Design review of the part built by this model. Coordinates are the model's own, in mm. Face numbers are marked on the shaded views. A direction names the side the tool comes from. Coordinates: 2 decimals unless noted, no trailing zeros. Write each loop counter-clockwise with the first axis right and the second up, starting at its lowest first coordinate (ties: lowest second). Pieces come first, ordered by that corner, then holes.
Q1. For pin 1 Ø4 at (x, z) = (-39.5, 0) entering from +Y, flat-tipped, find the tip position at first contact; note if it passes through.
Q2. The part is to be moulded in two halves that separate along X. For the marked faces 1, 2 and 3, say which applies: released by +X, released by -X, zero draft, split by the parting line, or undercut.
Q3. Take a section at A-A, the plane x = 39.5. Write out the cut boundary in (y, z) (3 decimals), plus the area to 3 significant figures.
Q4. Take a section at B-B, the plane y = 10.25. Write out the cut boundary in (x, z) (3 decimals), plus the area to 3 significant figures.
Q5. For L1, parallel to X at y = 4.75, z = 0 (3 decimals); L2, parallel to Z at x = -39.5, y = 3.75; L3, parallel to X at y = 8.75, z = -3 (3 decimals), list the stretches that pass through material, from the lowest coordinate up.
Q6. For the marked faces 4 and 5, list the 3-axis set-ups (+Z, -Z, +X, -X, +Y, -Y) from which the entire face can be reached by the end or side of a thin tool; tool diameter is ignored.
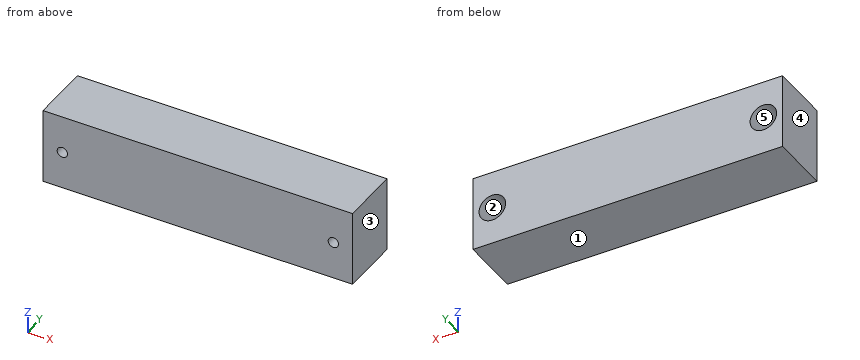
from build123d import *

# Parameters (mm, degrees)
SKETCH1_W               = 90.25
SKETCH1_H               = 22
BOSS_EXTRUDE1_DEPTH     = 17.5
SKETCH2_R               = 1.5
CUT_EXTRUDE1_DEPTH      = 1
CUT_EXTRUDE1_DEPTH_BACK = 18.5
SKETCH3_R               = 3.865
SKETCH3_R_2             = 1.5
CUT_EXTRUDE2_DEPTH      = 10


with BuildPart() as part:
    # Sketch1 → Boss-Extrude1 (new body)
    with BuildSketch(Plane(origin=(0, 0, 0), x_dir=(1, 0, 0), z_dir=(0, 1, 0))):
        Rectangle(SKETCH1_W, SKETCH1_H)
    extrude(amount=BOSS_EXTRUDE1_DEPTH)

    # Sketch2 → Cut-Extrude1 (cut, two sides)
    with BuildSketch(Plane(origin=(0, 17.5, 0), x_dir=(1, 0, 0), z_dir=(0, 1, 0))) as cut_extrude1_sk:
        with Locations((-39.5, 0)):
            Circle(SKETCH2_R)
        with Locations((39.5, 0)):
            Circle(SKETCH2_R)
    extrude(amount=CUT_EXTRUDE1_DEPTH, mode=Mode.SUBTRACT)
    extrude(cut_extrude1_sk.sketch, amount=-CUT_EXTRUDE1_DEPTH_BACK, mode=Mode.SUBTRACT)

    # Sketch3 → Cut-Extrude2 (cut)
    with BuildSketch(Plane(origin=(0, 17.5, 0), x_dir=(1, 0, 0), z_dir=(0, 1, 0))):
        with Locations((-39.5, 0)):
            Circle(SKETCH3_R)
        with Locations((-39.5, 0)):
            Circle(SKETCH3_R_2, mode=Mode.SUBTRACT)
        with Locations((39.5, 0)):
            Circle(SKETCH3_R)
        with Locations((39.5, 0)):
            Circle(SKETCH3_R_2, mode=Mode.SUBTRACT)
    extrude(amount=-CUT_EXTRUDE2_DEPTH, mode=Mode.SUBTRACT)


solid = part.part
Responses:
1. pin 1: stops at y = 7.5
2. face 1: zero draft
2. face 2: undercut
2. face 3: released by +X
3. outline: (0, -11) - (17.5, -11) - (17.5, -3.865) - (7.5, -3.865) - (7.5, -1.5) - (0, -1.5) - close; (0, 1.5) - (7.5, 1.5) - (7.5, 3.865) - (17.5, 3.865) - (17.5, 11) - (0, 11) - close
3. area: 285 mm2
4. outline: (-45.125, -11) - (45.125, -11) - (45.125, 11) - (-45.125, 11) - close; hole circle Ø7.73 at (-39.5, 0); hole circle Ø7.73 at (39.5, 0)
4. area: 1,890 mm2
5. L1: x = -45.125 to -41, -38 to 38, 41 to 45.125
5. L2: z = -11 to -1.5, 1.5 to 11
5. L3: x = -45.125 to -41.937, -37.063 to 37.063, 41.937 to 45.125
6. face 4: +Z, -Z, -X, +Y, -Y
6. face 5: +Y
